Design review of the part built by this model. Coordinates are the model's own, in mm. Face numbers are marked on the shaded views. A direction names the side the tool comes from. Coordinates: 2 decimals unless noted, no trailing zeros. Loops run counter-clockwise (first coordinate to the right, second up) from the corner with the lowest first, then second, coordinate; pieces in that order, holes last. Notation, with made-up numbers: (26, -5) -> (58, -5) arc R16 cw to (58, 15) -> close; hole circle Ø5 at (-36.5, 59). An arc over 180 degrees is marked (long way). One line per item, written item: value. Start each with the question number.
1. Add section B-B on z = -20.5. Write out the cut boundary in (x, y), plus the area to 3 significant figures.
2. Draft analysis for pull direction X (two halves, no side actions). For the marked faces 4, 5 and 6, state which applies: pulls with the +X half, pulls with the -X half, needs draft (parallel to the pull), parting line crosses it, or undercut.
3. Add section C-C on y = -1. Write out the cut boundary in (x, z), plus the area to 3 significant figures.
4. Add section A-A on x = -71. Write out the cut boundary in (y, z).
5. For probe 1 along Z at (x, y) = (-60, -1.5); probe 2 along Z at (x, y) = (-45.5, 53.5); probe 3 along X at (y, z) = (68.5, -38), list the stretches that pass through material, from the lowest coordinate up.
6. Machinability: for the marked faces 1, 2 and 3, which of the approach directions +Z, -Z, +X, -X, +Y, -Y give a long, thin tool a straight path to every point of the face, cutting with its end or side? Answer none if there is none.
7. Insertion check: pin 1 (6 mm diameter, centred on x = -49.5, z = -24.5, fed in from -Y). The pin has a flat end and moves straight along its axis. Give the tip position at first contact, or say it passes through.
```python
from build123d import *

# Parameters (mm, degrees)
SKETCH1_W            = 36
SKETCH1_H            = 36
SKETCH1_W_2          = 32
SKETCH1_H_2          = 32
BOSS_EXTRUDE1_DEPTH  = 10
SKETCH5_W            = 36
SKETCH5_H            = 36
SKETCH5_W_2          = 32
SKETCH5_H_2          = 32
BOSS_EXTRUDE5_DEPTH  = 63.5
SKETCH2_W            = 36
SKETCH2_H            = 36
SKETCH2_W_2          = 28
SKETCH2_H_2          = 28
BOSS_EXTRUDE9_DEPTH  = 2
SKETCH9_W            = 36
SKETCH9_H            = 36
SKETCH9_W_2          = 32
SKETCH9_H_2          = 32
BOSS_EXTRUDE11_DEPTH = 10


with BuildPart() as part:
    # Sketch1 → Boss-Extrude1 (new body)
    with BuildSketch(Plane(origin=(0, 0, 0), x_dir=(1, 0, 0), z_dir=(0, 1, 0))):
        with Locations((-61.04447382, 32.009277239)):
            Rectangle(SKETCH1_W, SKETCH1_H)
        with Locations((-61.04447382, 32.009277239)):
            Rectangle(SKETCH1_W_2, SKETCH1_H_2, mode=Mode.SUBTRACT)
    extrude(amount=BOSS_EXTRUDE1_DEPTH)

    # Sketch5 → Boss-Extrude5 (add)
    with BuildSketch(Plane(origin=(0, 10, 0), x_dir=(1, 0, 0), z_dir=(0, 1, 0))):
        with Locations((-61.04447382, 32.009277239)):
            Rectangle(SKETCH5_W, SKETCH5_H)
        with Locations((-61.04447382, 32.009277239)):
            Rectangle(SKETCH5_W_2, SKETCH5_H_2, mode=Mode.SUBTRACT)
    extrude(amount=BOSS_EXTRUDE5_DEPTH)

    # Sketch2 → Boss-Extrude9 (add)
    with BuildSketch(Plane.XZ):
        with Locations((-61.04447382, -32.009277239)):
            Rectangle(SKETCH2_W, SKETCH2_H)
        with Locations((-61.04447382, -32.009277239)):
            Rectangle(SKETCH2_W_2, SKETCH2_H_2, mode=Mode.SUBTRACT)
    extrude(amount=BOSS_EXTRUDE9_DEPTH)

    # Sketch9 → Boss-Extrude11 (add)
    with BuildSketch(Plane.XZ.offset(2)):
        with Locations((-61.04447382, -32.009277239)):
            Rectangle(SKETCH9_W, SKETCH9_H)
        with Locations((-61.04447382, -32.009277239)):
            Rectangle(SKETCH9_W_2, SKETCH9_H_2, mode=Mode.SUBTRACT)
    extrude(amount=BOSS_EXTRUDE11_DEPTH)


solid = part.part
```
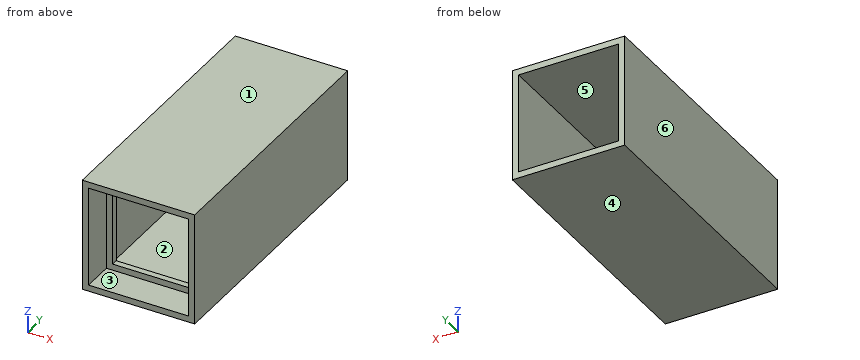
Worked answers:
1. outline: (-79.04, -12) -> (-77.04, -12) -> (-77.04, -2) -> (-75.04, -2) -> (-75.04, 0) -> (-77.04, 0) -> (-77.04, 73.5) -> (-79.04, 73.5) -> close; (-47.04, -2) -> (-45.04, -2) -> (-45.04, -12) -> (-43.04, -12) -> (-43.04, 73.5) -> (-45.04, 73.5) -> (-45.04, 0) -> (-47.04, 0) -> close
1. area: 350 mm²
2. face 4: needs draft
2. face 5: undercut
2. face 6: pulls with the -X half
3. outline: (-79.04, -50.01) -> (-43.04, -50.01) -> (-43.04, -14.01) -> (-79.04, -14.01) -> close; hole (-75.04, -46.01) -> (-47.04, -46.01) -> (-47.04, -18.01) -> (-75.04, -18.01) -> close
3. area: 512 mm²
4. outline: (-12, -50.01) -> (73.5, -50.01) -> (73.5, -48.01) -> (0, -48.01) -> (0, -46.01) -> (-2, -46.01) -> (-2, -48.01) -> (-12, -48.01) -> close; (-12, -16.01) -> (-2, -16.01) -> (-2, -18.01) -> (0, -18.01) -> (0, -16.01) -> (73.5, -16.01) -> (73.5, -14.01) -> (-12, -14.01) -> close
5. probe 1: z = -50.01 to -46.01, -18.01 to -14.01
5. probe 2: z = -50.01 to -48.01, -16.01 to -14.01
5. probe 3: x = -79.04 to -77.04, -45.04 to -43.04
6. face 1: +Z, +X, -X, +Y, -Y
6. face 2: +Y
6. face 3: -Y
7. pin 1: stops at y = -2
